```python
from build123d import *

# Parameters (mm, degrees)
SKETCH1_W           = 80
SKETCH1_H           = 38.1
SKETCH1_R           = 5
SKETCH1_R_2         = 10.5
SKETCH1_R_3         = 3.5
BOSS_EXTRUDE1_DEPTH = 20
BOSS_EXTRUDE2_START = 10
SKETCH1_4_R         = 10.5
SKETCH1_4_R_2       = 5.25
BOSS_EXTRUDE2_DEPTH = 10
BOSS_EXTRUDE4_START = -5
SKETCH1_6_W         = 80
SKETCH1_6_H         = 38.1
SKETCH1_6_R         = 5
SKETCH1_6_R_2       = 10.5
SKETCH1_6_R_3       = 3.5
BOSS_EXTRUDE4_DEPTH = 5
FILLET2_R           = 1
SKETCH3_R           = 3.5
CUT_EXTRUDE1_DEPTH  = 10


with BuildPart() as part:
    # Sketch1 → Boss-Extrude1 (new body)
    # profile 1 of 3: a face of its own
    with BuildSketch(Plane(origin=(0, 0, 0), x_dir=(1, 0, 0), z_dir=(0, 1, 0))):
        with Locations((40, -19.05)):
            Rectangle(SKETCH1_W, SKETCH1_H)
        with Locations((70, -19.05)):
            Circle(SKETCH1_R, mode=Mode.SUBTRACT)
        with Locations((10, -19.05)):
            Circle(SKETCH1_R, mode=Mode.SUBTRACT)
        with Locations(Location((40, -19.05, 0), (0, 0, 270))):
            Circle(SKETCH1_R_2, mode=Mode.SUBTRACT)
    # profile 2 of 3: a face of its own
    with BuildSketch(Plane(origin=(0, 0, 0), x_dir=(1, 0, 0), z_dir=(0, 1, 0))):
        with Locations((10, -19.05)):
            Circle(SKETCH1_R)
        with Locations(Location((10, -19.05, 0), (0, 0, 270))):
            Circle(SKETCH1_R_3, mode=Mode.SUBTRACT)
    # profile 3 of 3: a face of its own
    with BuildSketch(Plane(origin=(0, 0, 0), x_dir=(1, 0, 0), z_dir=(0, 1, 0))):
        with Locations((70, -19.05)):
            Circle(SKETCH1_R)
        with Locations(Location((70, -19.05, 0), (0, 0, 270))):
            Circle(SKETCH1_R_3, mode=Mode.SUBTRACT)
    extrude(amount=BOSS_EXTRUDE1_DEPTH)

    # Sketch1<4> → Boss-Extrude2 (add)
    with BuildSketch(Plane(origin=(0, 0, 0), x_dir=(1, 0, 0), z_dir=(0, 1, 0)).offset(BOSS_EXTRUDE2_START)):
        with Locations(Location((40, -19.05, 0), (0, 0, 270))):
            Circle(SKETCH1_4_R)
        with Locations(Location((40, -19.05, 0), (0, 0, 270))):
            Circle(SKETCH1_4_R_2, mode=Mode.SUBTRACT)
    extrude(amount=BOSS_EXTRUDE2_DEPTH)

    # Sketch1<6> → Boss-Extrude4 (add)
    # profile 1 of 3: a face of its own
    with BuildSketch(Plane(origin=(0, 0, 0), x_dir=(1, 0, 0), z_dir=(0, 1, 0)).offset(BOSS_EXTRUDE4_START)):
        with Locations((40, -19.05)):
            Rectangle(SKETCH1_6_W, SKETCH1_6_H)
        with Locations((70, -19.05)):
            Circle(SKETCH1_6_R, mode=Mode.SUBTRACT)
        with Locations((10, -19.05)):
            Circle(SKETCH1_6_R, mode=Mode.SUBTRACT)
        with Locations(Location((40, -19.05, 0), (0, 0, 270))):
            Circle(SKETCH1_6_R_2, mode=Mode.SUBTRACT)
    # profile 2 of 3: a face of its own
    with BuildSketch(Plane(origin=(0, 0, 0), x_dir=(1, 0, 0), z_dir=(0, 1, 0)).offset(BOSS_EXTRUDE4_START)):
        with Locations((70, -19.05)):
            Circle(SKETCH1_6_R)
        with Locations(Location((70, -19.05, 0), (0, 0, 270))):
            Circle(SKETCH1_6_R_3, mode=Mode.SUBTRACT)
    # profile 3 of 3: a face of its own
    with BuildSketch(Plane(origin=(0, 0, 0), x_dir=(1, 0, 0), z_dir=(0, 1, 0)).offset(BOSS_EXTRUDE4_START)):
        with Locations((10, -19.05)):
            Circle(SKETCH1_6_R)
        with Locations(Location((10, -19.05, 0), (0, 0, 270))):
            Circle(SKETCH1_6_R_3, mode=Mode.SUBTRACT)
    extrude(amount=BOSS_EXTRUDE4_DEPTH)

    # Fillet2
    fillet2_edges = [part.edges().sort_by_distance(p)[0] for p in [
        (80, 20, 19.05),
        (80, 7.5, 38.1),
        (0, 7.5, 38.1),
        (0, 7.5, 0),
        (80, 7.5, 0),
        (40, 20, 0),
        (0, 20, 19.05),
        (40, 20, 13.8),
        (40, 20, 38.1),
        (40, -5, 38.1),
        (0, -5, 19.05),
        (40, -5, 8.55),
        (10, 20, 15.55),
        (80, -5, 19.05),
        (40, -5, 0),
        (70, 20, 15.55),
    ]]
    fillet(fillet2_edges, radius=FILLET2_R)

    # Sketch3 → Cut-Extrude1 (cut)
    with BuildSketch(Plane.XY):
        with Locations((40, 5.5)):
            Circle(SKETCH3_R)
        with Locations((40, 2)):
            Circle(SKETCH3_R)
        with BuildLine():
            ThreePointArc((43.031088913, 3.75), (43.380740392, 2.905866658), (43.5, 2))
            Line((43.5, 2), (43.5, 5.5))
            ThreePointArc((43.5, 5.5), (43.380740392, 4.594133342), (43.031088913, 3.75))
        make_face()
        with BuildLine():
            Line((36.5, 5.5), (36.5, 2))
            ThreePointArc((36.5, 2), (36.619259608, 2.905866658), (36.968911087, 3.75))
            ThreePointArc((36.968911087, 3.75), (36.619259608, 4.594133342), (36.5, 5.5))
        make_face()
    extrude(amount=CUT_EXTRUDE1_DEPTH, mode=Mode.SUBTRACT)


solid = part.part
```
Work out the finished part from the listing and answer in its coordinate system (mm). A direction names the side the tool comes from. Round coordinates to 2 decimals unless told otherwise and drop trailing zeros. Write each loop counter-clockwise with the first axis right and the second up, starting at its lowest first coordinate (ties: lowest second). Pieces come first, ordered by that corner, then holes.
1) A flat-ended cylindrical pin translates along its axis: P1, Ø12, axis at x = 40, z = 19.05, coming from the -Y side. Find the tip coordinate at first contact, or state that the pin passes through.
2) A cutting plane is placed at D-D on y = 15. Determine the outline of the cut face in (x, z).
3) A cutting plane is placed at B-B on x = 70. Determine the outline of the cut face in (y, z).
4) Consider probe 1 along X at (y, z) = (2.75, 19); probe 2 along X at (y, z) = (-3, 22); probe 3 along X at (y, z) = (8.5, 4). Determine where each line is inside the solid, lowest interval first.
5) Which of the six approach directions +Z, -Z, +X, -X, +Y, -Y give full straight-line access (tool end or side, diameter ignored) to faces 1 (the face through (38, 10, 14)), 2 (the face through (41, 20, 11)), 3 (the face through (36.5, 4, 5))?
6) A cutting plane is placed at A-A on x = 40. Determine the outline of the cut face in (y, z), and give its area (3 significant figures).
7) A cutting plane is placed at C-C on z = 19.05. Give the number of separate pieces and of enclosed holes in the cut face, and give its area (3 significant figures).
8) Determine the mould class of faces 4 (the face through (80, 7, 19)), 5 (the face through (6.895, 6.832, 20.665)), 6 (the face through (39, 10, 0)) for opening direction X: pulls with the +X half, pulls with the -X half, needs draft (parallel to the pull), parting line crosses it, or undercut.
Entries:
1. P1: stops at y = 10
2. outline: (0, 1) arc R1 ccw to (1, 0) - (79, 0) arc R1 ccw to (80, 1) - (80, 37.1) arc R1 ccw to (79, 38.1) - (1, 38.1) arc R1 ccw to (0, 37.1) - close; hole circle Ø7 at (10, 19.05); hole circle Ø10.5 at (40, 19.05); hole circle Ø7 at (70, 19.05)
3. outline: (-5, 1) arc R1 ccw to (-4, 0) - (19, 0) arc R1 ccw to (20, 1) - (20, 14.55) arc R1 ccw to (19, 15.55) - (-5, 15.55) - close; (-5, 22.55) - (19, 22.55) arc R1 ccw to (20, 23.55) - (20, 37.1) arc R1 ccw to (19, 38.1) - (-4, 38.1) arc R1 ccw to (-5, 37.1) - close
4. probe 1: x = 0 to 6.5, 13.5 to 29.5, 50.5 to 66.5, 73.5 to 80
4. probe 2: x = 0 to 8.12, 11.88 to 29.92, 50.08 to 68.12, 71.88 to 80
4. probe 3: x = 0 to 38.2, 41.8 to 80
5. face 1: -Y
5. face 2: +Z, -Z, +X, -X, +Y
5. face 3: -Z
6. outline: (-5, 1) arc R1 ccw to (-4, 0) - (-1.5, 0) - (-1.5, 8.55) - (-4, 8.55) arc R1 ccw to (-5, 7.55) - close; (-5, 30.55) arc R1 ccw to (-4, 29.55) - (10, 29.55) - (10, 24.3) - (19, 24.3) arc R1 ccw to (20, 25.3) - (20, 37.1) arc R1 ccw to (19, 38.1) - (-4, 38.1) arc R1 ccw to (-5, 37.1) - close; (9, 0) - (19, 0) arc R1 ccw to (20, 1) - (20, 12.8) arc R1 ccw to (19, 13.8) - (10, 13.8) - (10, 8.55) - (9, 8.55) - close
6. area: 441 mm2
7. separate pieces: 4
7. enclosed holes: 0
7. area: 1,230 mm2
8. face 4: pulls with the +X half
8. face 5: undercut
8. face 6: needs draft
